```python
from build123d import *

# Parameters (mm, degrees)
SKETCH1_W           = 45
SKETCH1_H           = 40
BOSS_EXTRUDE1_DEPTH = 6
SKETCH2_W           = 5
SKETCH2_H           = 5
SKETCH2_H_2         = 7
CUT_EXTRUDE1_DEPTH  = 6
SKETCH3_W           = 5
SKETCH3_H           = 5
SKETCH3_H_2         = 3
SKETCH3_H_3         = 10
CUT_EXTRUDE2_DEPTH  = 6
SKETCH4_W           = 5
SKETCH4_H           = 25
BOSS_EXTRUDE3_DEPTH = 6
SKETCH8_W           = 5
SKETCH8_H           = 5
CUT_EXTRUDE5_DEPTH  = 6
SKETCH9_W           = 5
SKETCH9_H           = 40
BOSS_EXTRUDE4_DEPTH = 6
SKETCH10_W          = 5
SKETCH10_H          = 5
SKETCH10_H_2        = 3
SKETCH10_H_3        = 10
CUT_EXTRUDE7_DEPTH  = 6


with BuildPart() as part:
    # Sketch1 → Boss-Extrude1 (new body)
    with BuildSketch(Plane.XY):
        with Locations((1.238898757, -2.615452931)):
            Rectangle(SKETCH1_W, SKETCH1_H)
    extrude(amount=BOSS_EXTRUDE1_DEPTH)

    # Sketch2 → Cut-Extrude1 (cut)
    with BuildSketch(Plane.XY.offset(6)):
        with Locations((-18.761101243, 4.884547069)):
            Rectangle(SKETCH2_W, SKETCH2_H)
        with Locations((-18.761101243, -4.115452931)):
            Rectangle(SKETCH2_W, SKETCH2_H_2)
        with Locations((-18.761101243, -15.115452931)):
            Rectangle(SKETCH2_W, SKETCH2_H)
    extrude(amount=-CUT_EXTRUDE1_DEPTH, mode=Mode.SUBTRACT)

    # Sketch3 → Cut-Extrude2 (cut)
    with BuildSketch(Plane.XY.offset(6)):
        with Locations((21.238898757, -20.115452931)):
            Rectangle(SKETCH3_W, SKETCH3_H)
        with Locations((21.238898757, -9.115452931)):
            Rectangle(SKETCH3_W, SKETCH3_H_2)
        with Locations((21.238898757, 14.884547069)):
            Rectangle(SKETCH3_W, SKETCH3_H)
        with Locations((21.238898757, 2.384547069)):
            Rectangle(SKETCH3_W, SKETCH3_H_3)
    extrude(amount=-CUT_EXTRUDE2_DEPTH, mode=Mode.SUBTRACT)

    # Sketch4 → Boss-Extrude3 (add)
    with BuildSketch(Plane.XY.offset(6)):
        with Locations((-18.761101243, -5.115452931)):
            Rectangle(SKETCH4_W, SKETCH4_H)
    extrude(amount=-BOSS_EXTRUDE3_DEPTH)

    # Sketch8 → Cut-Extrude5 (cut)
    with BuildSketch(Plane.XY.offset(6)):
        with Locations((-18.761101243, -5.115452931)):
            Rectangle(SKETCH8_W, SKETCH8_H)
        with Locations((-18.761101243, -13.115452931)):
            Rectangle(SKETCH8_W, SKETCH8_H)
        with Locations((-18.761101243, 9.884547069)):
            Rectangle(SKETCH8_W, SKETCH8_H)
    extrude(amount=-CUT_EXTRUDE5_DEPTH, mode=Mode.SUBTRACT)

    # Sketch9 → Boss-Extrude4 (add)
    with BuildSketch(Plane.XY.offset(6)):
        with Locations((21.238898757, -2.615452931)):
            Rectangle(SKETCH9_W, SKETCH9_H)
    extrude(amount=-BOSS_EXTRUDE4_DEPTH)

    # Sketch10 → Cut-Extrude7 (cut)
    with BuildSketch(Plane.XY.offset(6)):
        with Locations((21.238898757, 14.884547069)):
            Rectangle(SKETCH10_W, SKETCH10_H)
        with Locations((21.238898757, 4.884547069)):
            Rectangle(SKETCH10_W, SKETCH10_H)
        with Locations((21.238898757, -6.115452931)):
            Rectangle(SKETCH10_W, SKETCH10_H_2)
        with Locations((21.238898757, -17.615452931)):
            Rectangle(SKETCH10_W, SKETCH10_H_3)
    extrude(amount=-CUT_EXTRUDE7_DEPTH, mode=Mode.SUBTRACT)


solid = part.part
```
Design review of the part built by this model. Coordinates are the model's own, in mm. A direction names the side the tool comes from. Give positions to 0.01 mm unless a question says otherwise; leave off trailing zeros. Write each loop counter-clockwise with the first axis right and the second up, starting at its lowest first coordinate (ties: lowest second). Pieces come first, ordered by that corner, then holes.
(1) Clearance check with flat-ended pins moving along their axes: pin 1 Ø1.5 at (x, z) = (20.5, 3.5) entering from -Y; pin 2 Ø1.5 at (y, z) = (5.5, 2.5) entering from +X; pin 3 Ø1.5 at (y, z) = (-4.5, 2.5) entering from -X. State where each tip first meets the part, or that it passes through.
Checked values:
pin 1: stops at y = -12.62
pin 2: stops at x = 18.74
pin 3: stops at x = -16.26
(2) Mouldability with a two-part tool opening along Y and no side actions: class faces 1 (the face through (-16.261, -5, 3)), 2 (the face through (21, 12.385, 3)), 3 (the face through (-2, -22.615, 3)), 4 (the face through (23.739, -10, 3)) as +Y half, -Y half, draft (parallel to the pull), parting line (faces both ways), or undercut.
Checked values:
face 1: undercut
face 2: +Y half
face 3: -Y half
face 4: draft
(3) Wall thickness on line 1 along Y through (x, z) = (-17, 2.4); line 2 along X through (y, z) = (-11, 4.55); line 3 along X through (y, z) = (-20, 4.35): over which ranges is each line inside the solid? List them lowest first.
Checked values:
line 1: y = -22.62 to -15.62, -10.62 to -7.62, -2.62 to 7.38, 12.38 to 17.38
line 2: x = -16.26 to 23.74
line 3: x = -21.26 to 18.74
(4) Add section B-B (z = 3.9). Give the boundary of the cut face in (x, y), and give its area (3 significant figures).
Checked values:
outline: (-21.26, -22.62) - (18.74, -22.62) - (18.74, -12.62) - (23.74, -12.62) - (23.74, -7.62) - (18.74, -7.62) - (18.74, -4.62) - (23.74, -4.62) - (23.74, 2.38) - (18.74, 2.38) - (18.74, 7.38) - (23.74, 7.38) - (23.74, 12.38) - (18.74, 12.38) - (18.74, 17.38) - (-21.26, 17.38) - (-21.26, 12.38) - (-16.26, 12.38) - (-16.26, 7.38) - (-21.26, 7.38) - (-21.26, -2.62) - (-16.26, -2.62) - (-16.26, -7.62) - (-21.26, -7.62) - (-21.26, -10.62) - (-16.26, -10.62) - (-16.26, -15.62) - (-21.26, -15.62) - close
area: 1,610 mm2
(5) Tool access review of faces 5 (the face through (21, -7.615, 3)), 6 (the face through (-19, -10.615, 3)), 7 (the face through (18.739, 15, 3)), 8 (the face through (23.739, -1, 3)): name each direction out of +Z, -Z, +X, -X, +Y, -Y from which nothing blocks a thin tool from reaching the whole face with its end or side.
Checked values:
face 5: +Z, -Z, +X
face 6: +Z, -Z, -X
face 7: +Z, -Z, +X, +Y
face 8: +Z, -Z, +X, +Y, -Y
(6) Add section A-A (x = -17). Give the boundary of the cut face in (y, z), and give its area (3 significant figures).
Checked values:
outline: (-22.62, 0) - (-15.62, 0) - (-15.62, 6) - (-22.62, 6) - close; (-10.62, 0) - (-7.62, 0) - (-7.62, 6) - (-10.62, 6) - close; (-2.62, 0) - (7.38, 0) - (7.38, 6) - (-2.62, 6) - close; (12.38, 0) - (17.38, 0) - (17.38, 6) - (12.38, 6) - close
area: 150 mm2
(7) Add section C-C (y = -3.5). Give the boundary of the cut face in (x, z), and give its area (3 significant figures).
Checked values:
outline: (-16.26, 0) - (23.74, 0) - (23.74, 6) - (-16.26, 6) - close
area: 240 mm2
(8) Add section D-D (y = -15). Give the boundary of the cut face in (x, z).
Checked values:
outline: (-16.26, 0) - (18.74, 0) - (18.74, 6) - (-16.26, 6) - close
